Geometry: final body of the model. Coordinates: model frame, mm. Round coordinates to 2 decimals unless told otherwise and drop trailing zeros. Order: outer loops, then holes, each group sorted by start corner. A loop starts at its lowest first (then second) coordinate and runs counter-clockwise, first axis right, second up. Notation, with made-up numbers: (6.5, 86.5) - (47.5, 86.5) arc R21 cw to (47.5, 113.5) - close; hole circle Ø9 at (71.5, -28). An arc over 180 degrees is marked (long way). Put each result on its own line as item: value. Start each with the question number.
(1) Section A-A (x = 28). Output: boundary loops of the cut face in (y, z), and give its area (3 significant figures).
(2) Material intervals for L1, parallel to Y at x = -15, z = 0.7; L2, parallel to X at y = 2, z = 0.7; L3, parallel to X at y = 4.5, z = 0.2, sorted ascending. Write a range as [from, to].
(3) Section B-B (y = -5). Output: boundary loops of the cut face in (x, z), and give its area (3 significant figures).
(4) Section D-D (x = 5). Output: boundary loops of the cut face in (y, z), and give its area (3 significant figures).
(5) Pin query (flat end, axial travel): P1, Ø0.5, axis at x = 14.5, z = 0.5, coming from the +Y side. Return the tip coordinate at first contact, or that it passes through.
(6) Section C-C (z = 0.25). Output: boundary loops of the cut face in (x, y), and give its area (3 significant figures).
from build123d import *

# Parameters (mm, degrees)
SKETCH_1_R      = 1.25
EXTRUDE_1_DEPTH = 1


with BuildPart() as part:
    # 草图1 → 凸台-拉伸1 (new body)
    with BuildSketch(Plane.XY):
        with BuildLine():
            Line((41, -7.95), (41, 7.95))
            ThreePointArc((41, 7.95), (39.242640687, 12.192640687), (35, 13.95))
            Line((35, 13.95), (-15, 11.95))
            ThreePointArc((-15, 11.95), (-17.828427125, 10.778427125), (-19, 7.95))
            Line((-19, 7.95), (-19, -7.95))
            ThreePointArc((-19, -7.95), (-17.828427125, -10.778427125), (-15, -11.95))
            Line((-15, -11.95), (35, -13.95))
            ThreePointArc((35, -13.95), (39.242640687, -12.192640687), (41, -7.95))
        make_face()
        with Locations((35, -5)):
            Circle(SKETCH_1_R, mode=Mode.SUBTRACT)
        with Locations((35, 5)):
            Circle(SKETCH_1_R, mode=Mode.SUBTRACT)
        with Locations((-15, -5)):
            Circle(SKETCH_1_R, mode=Mode.SUBTRACT)
        with Locations((-15, 5)):
            Circle(SKETCH_1_R, mode=Mode.SUBTRACT)
        with BuildLine():
            Line((29.75, 10.85), (-9.75, 10.85))
            ThreePointArc((-9.75, 10.85), (-10.739949494, 10.439949494), (-11.15, 9.45))
            Line((-11.15, 9.45), (-11.15, -9.45))
            ThreePointArc((-11.15, -9.45), (-10.739949494, -10.439949494), (-9.75, -10.85))
            Line((-9.75, -10.85), (29.75, -10.85))
            ThreePointArc((29.75, -10.85), (30.739949494, -10.439949494), (31.15, -9.45))
            Line((31.15, -9.45), (31.15, 9.45))
            ThreePointArc((31.15, 9.45), (30.739949494, 10.439949494), (29.75, 10.85))
        make_face(mode=Mode.SUBTRACT)
    extrude(amount=EXTRUDE_1_DEPTH)


solid = part.part
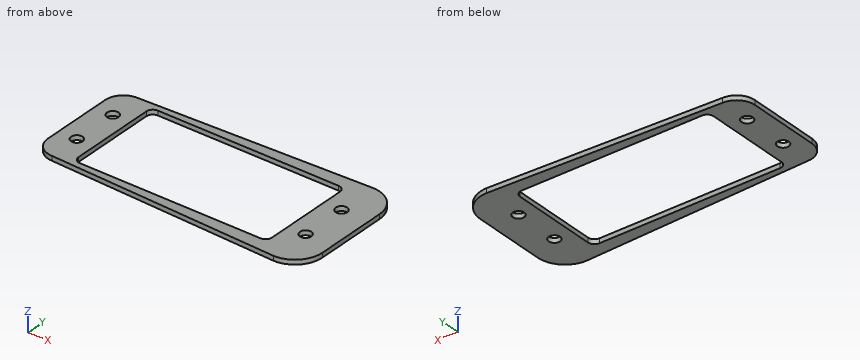
Checks:
1. outline: (-13.67, 0) - (-10.85, 0) - (-10.85, 1) - (-13.67, 1) - close; (10.85, 0) - (13.67, 0) - (13.67, 1) - (10.85, 1) - close
1. area: 5.64 mm²
2. L1: y = [-11.95, -6.25], [-3.75, 3.75], [6.25, 11.95]
2. L2: x = [-19, -11.15], [31.15, 41]
2. L3: x = [-19, -16.15], [-13.85, -11.15], [31.15, 33.85], [36.15, 41]
3. outline: (-19, 0) - (-16.25, 0) - (-16.25, 1) - (-19, 1) - close; (-13.75, 0) - (-11.15, 0) - (-11.15, 1) - (-13.75, 1) - close; (31.15, 0) - (33.75, 0) - (33.75, 1) - (31.15, 1) - close; (36.25, 0) - (41, 0) - (41, 1) - (36.25, 1) - close
3. area: 12.7 mm²
4. outline: (-12.75, 0) - (-10.85, 0) - (-10.85, 1) - (-12.75, 1) - close; (10.85, 0) - (12.75, 0) - (12.75, 1) - (10.85, 1) - close
4. area: 3.80 mm²
5. P1: stops at y = 13.14
6. outline: (-19, -7.95) arc R4 ccw to (-15, -11.95) - (35, -13.95) arc R6 ccw to (41, -7.95) - (41, 7.95) arc R6 ccw to (35, 13.95) - (-15, 11.95) arc R4 ccw to (-19, 7.95) - close; hole circle Ø2.5 at (-15, -5); hole circle Ø2.5 at (-15, 5); hole (-11.15, -9.45) arc R1.4 ccw to (-9.75, -10.85) - (29.75, -10.85) arc R1.4 ccw to (31.15, -9.45) - (31.15, 9.45) arc R1.4 ccw to (29.75, 10.85) - (-9.75, 10.85) arc R1.4 ccw to (-11.15, 9.45) - close; hole circle Ø2.5 at (35, -5); hole circle Ø2.5 at (35, 5)
6. area: 600 mm²
